Job drawing, mm, ordinate dimensions from the low corner. One solid piece. A direction names the side the tool comes from. Give positions to 0.01 mm unless a question says otherwise; leave off trailing zeros. Order: outer loops, then holes, each group sorted by start corner. A loop starts at its lowest first (then second) coordinate and runs counter-clockwise, first axis right, second up. Notation, with made-up numbers: M 36,-37.5 L 84,-37.5 A18 cw 84,-6.5 Z; hole C 0.5,62 d3. An arc over 180 degrees is marked long. One line per item, written item: value. Start each with the question number.
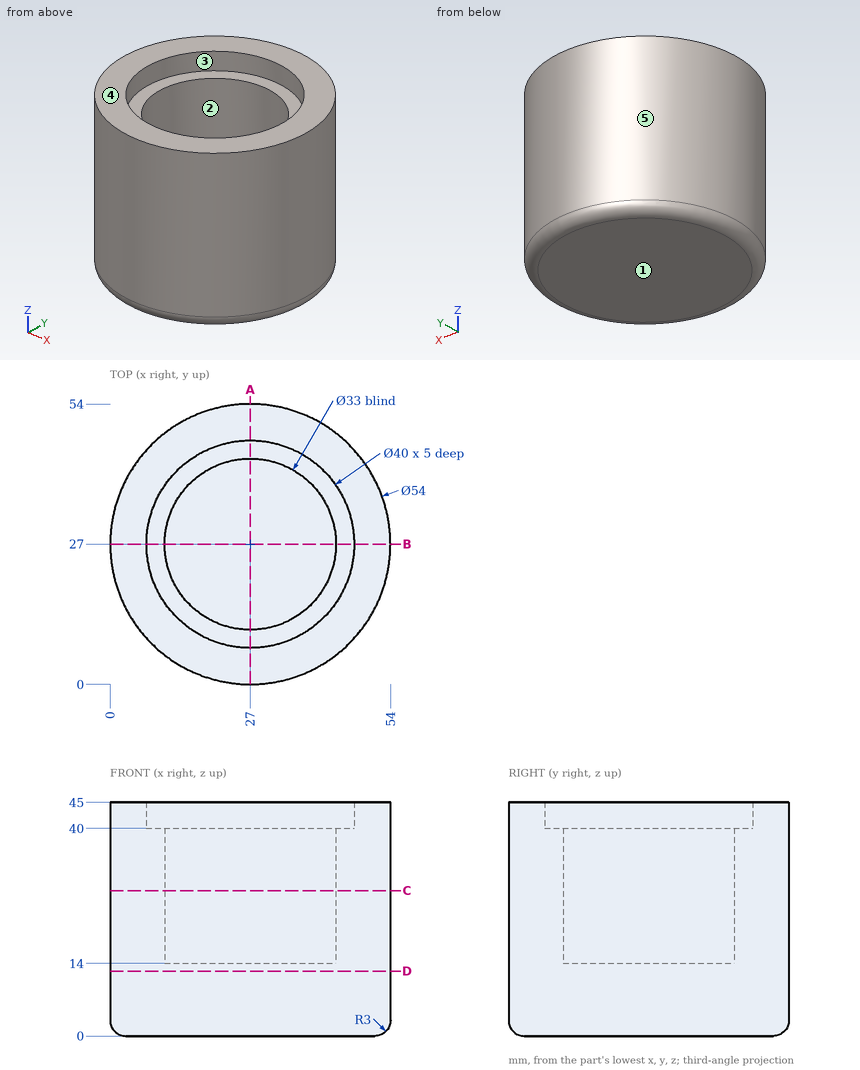
1) Tool access for the marked faces 1 and 2: list every direction of +Z, -Z, +X, -X, +Y, -Y with a clear straight run to the whole face (end or side of a thin tool).
2) Drill centre lines: line 1 (Z direction, x = 38.5, y = 41.5); line 2 (Y direction, x = 27, z = 23.25); line 3 (Z direction, x = 45.5, y = 42.5). Where is each one in solid material? Low to high.
3) Drop flat-ended pins along their axis: P1, Ø16.5, axis at x = 25.5, y = 26.5, coming from the +Z side; P2, Ø6, axis at y = 13.5, z = 33.5, coming from the -X side; P3, Ø1, axis at y = 34, z = 11, coming from the -X side. Give the stop position or say it passes through.
4) Slice it at C-C (z = 28). List the corners of the cut face in (x, y).
5) Slice it at D-D (z = 12.5). List the corners of the cut face in (x, y).
6) Slice it at A-A (x = 27). List the corners of the cut face in (y, z), plus the area to 3 significant figures.
7) Pull direction X, two halves, no side cores. Call the marked faces 3, 4 and 5: pulls with the +X half, pulls with the -X half, needs draft (parallel to the pull), parting line crosses it, or undercut.
Results list:
1. face 1: -Z, +X, -X, +Y, -Y
1. face 2: +Z
2. line 1: z = 0 to 40
2. line 2: y = 0 to 10.5, 43.5 to 54
2. line 3: z = 0 to 45
3. P1: stops at z = 14
3. P2: stops at x = 2.13
3. P3: stops at x = 0.79
4. outline: C 27,27 d54; hole C 27,27 d33
5. outline: C 27,27 d54
6. outline: M 0,3 A3 ccw 3,0 L 51,0 A3 ccw 54,3 L 54,45 L 47,45 L 47,40 L 43.5,40 L 43.5,14 L 10.5,14 L 10.5,40 L 7,40 L 7,45 L 0,45 Z
6. area: 1,370 mm²
7. face 3: undercut
7. face 4: needs draft
7. face 5: parting line crosses it
